```python
from build123d import *

# Parameters (mm, degrees)
SKETCH003_W     = 275
SKETCH003_H     = 100
PAD_DEPTH       = 6.35
SKETCH_R        = 3.25
POCKET_DEPTH    = 6.351
SKETCH004_R     = 3.25
POCKET001_DEPTH = 6.351
POCKET002_DEPTH = 6.351
SKETCH007_R     = 3.25
POCKET003_DEPTH = 6.351


with BuildPart() as part:
    # Sketch003 → Pad (new body)
    with BuildSketch(Plane(origin=(0, 0, 0), x_dir=(1, 0, 0), z_dir=(0, 0, -1))):
        with Locations((137.5, 50)):
            Rectangle(SKETCH003_W, SKETCH003_H)
    extrude(amount=PAD_DEPTH)

    # Sketch → Pocket (cut, through all)
    with BuildSketch(Plane.XY):
        with Locations((110, -12.5)):
            Circle(SKETCH_R)
        with Locations((165, -12.5)):
            Circle(SKETCH_R)
    extrude(amount=-POCKET_DEPTH, mode=Mode.SUBTRACT)

    # Sketch004 → Pocket001 (cut, through all)
    with BuildSketch(Plane.XY):
        with Locations((12.5, -12.5)):
            Circle(SKETCH004_R)
        with Locations((12.5, -67.5)):
            Circle(SKETCH004_R)
        with Locations((262.5, -12.5)):
            Circle(SKETCH004_R)
        with Locations((262.5, -67.5)):
            Circle(SKETCH004_R)
    extrude(amount=-POCKET001_DEPTH, mode=Mode.SUBTRACT)

    # Sketch005 → Pocket002 (cut, through all)
    with BuildSketch(Plane.XY):
        with BuildLine():
            ThreePointArc((112.2, -39.999985), (110, -37.8), (107.8, -39.999985))
            Line((107.8, -39.999985), (107.8, -55.999992))
            ThreePointArc((107.8, -55.999992), (110, -58.2), (112.2, -55.999992))
            Line((112.2, -39.999985), (112.2, -55.999992))
        make_face()
        with BuildLine():
            ThreePointArc((167.2, -39.999991), (165, -37.8), (162.8, -39.999991))
            Line((162.8, -39.999991), (162.8, -55.999999))
            ThreePointArc((162.8, -55.999999), (165, -58.2), (167.2, -55.999999))
            Line((167.2, -39.999991), (167.2, -55.999999))
        make_face()
    extrude(amount=-POCKET002_DEPTH, mode=Mode.SUBTRACT)

    # Sketch007 → Pocket003 (cut, through all)
    with BuildSketch(Plane.XY):
        with Locations((43.5, -30)):
            Circle(SKETCH007_R)
        with Locations((73.5, -30)):
            Circle(SKETCH007_R)
        with Locations((201.5, -30)):
            Circle(SKETCH007_R)
        with Locations((231.5, -30)):
            Circle(SKETCH007_R)
    extrude(amount=-POCKET003_DEPTH, mode=Mode.SUBTRACT)


solid = part.part
```
Geometry check sheet. Reference: the model listing, model coordinates, mm. A direction names the side the tool comes from. Round coordinates to 2 decimals unless told otherwise and drop trailing zeros. Order: outer loops, then holes, each group sorted by start corner. A loop starts at its lowest first (then second) coordinate and runs counter-clockwise, first axis right, second up. Notation, with made-up numbers: M -38,39 L -11,39 A19 ccw -11,71 Z; hole C -8,-40 d4. An arc over 180 degrees is marked long. Answer as CSV lines item,"result".
1) Mould release check, pull along Y, two halves, no side actions. Record for faces 3 (the face through (136, -51, 0)), 4 (the face through (136, -100, -3)), 5 (the face through (106.753, -12.357, -3.131)): +Y half, -Y half, draft (parallel to the pull), parting line (faces both ways), or undercut.
Entries:
face 3,"draft"
face 4,"-Y half"
face 5,"undercut"
2) Sectioned sample at C-C on z = -5.25. Give the number of separate pieces and of enclosed holes in the cut face, and give its area (3 significant figures).
Entries:
separate pieces,"1"
enclosed holes,"12"
area,"27,000 mm2"
3) Tool access check on faces 1 (the face through (136, 0, -3)), 2 (the face through (162.8, -48, -3)). Record the directions out of +Z, -Z, +X, -X, +Y, -Y that give a thin tool (end or side, any length) a straight path to the whole face; none if there is none.
Entries:
face 1,"+Z, -Z, +X, -X, +Y"
face 2,"+Z, -Z"
4) Sectioned sample at A-A on x = 231.5. Record the cut outline in (y, z), and give its area (3 significant figures).
Entries:
outline,"M -100,-6.35 L -33.25,-6.35 L -33.25,0 L -100,0 Z; M -26.75,-6.35 L 0,-6.35 L 0,0 L -26.75,0 Z"
area,"594 mm2"
5) Sectioned sample at B-B on y = -30. Record the cut outline in (x, z).
Entries:
outline,"M 0,-6.35 L 40.25,-6.35 L 40.25,0 L 0,0 Z; M 46.75,-6.35 L 70.25,-6.35 L 70.25,0 L 46.75,0 Z; M 76.75,-6.35 L 198.25,-6.35 L 198.25,0 L 76.75,0 Z; M 204.75,-6.35 L 228.25,-6.35 L 228.25,0 L 204.75,0 Z; M 234.75,-6.35 L 275,-6.35 L 275,0 L 234.75,0 Z"
6) Thickness scan on probe 1 along X at (y, z) = (-41.5, -2); probe 2 along X at (y, z) = (-29.5, -4.5); probe 3 along Y at (x, z) = (262.5, -3.25). Record the ranges inside material, lowest first. Write a range as [from, to].
Entries:
probe 1,"[0, 107.8], [112.2, 162.8], [167.2, 275]"
probe 2,"[0, 40.29], [46.71, 70.29], [76.71, 198.29], [204.71, 228.29], [234.71, 275]"
probe 3,"[-100, -70.75], [-64.25, -15.75], [-9.25, 0]"
7) Sectioned sample at D-D on x = 262.5. Record the cut outline in (y, z).
Entries:
outline,"M -100,-6.35 L -70.75,-6.35 L -70.75,0 L -100,0 Z; M -64.25,-6.35 L -15.75,-6.35 L -15.75,0 L -64.25,0 Z; M -9.25,-6.35 L 0,-6.35 L 0,0 L -9.25,0 Z"
